Read the model definition and answer for the solid it produces. Units are mm, in the model's axes. Face numbers are marked on the shaded views. Round coordinates to 2 decimals unless told otherwise and drop trailing zeros.
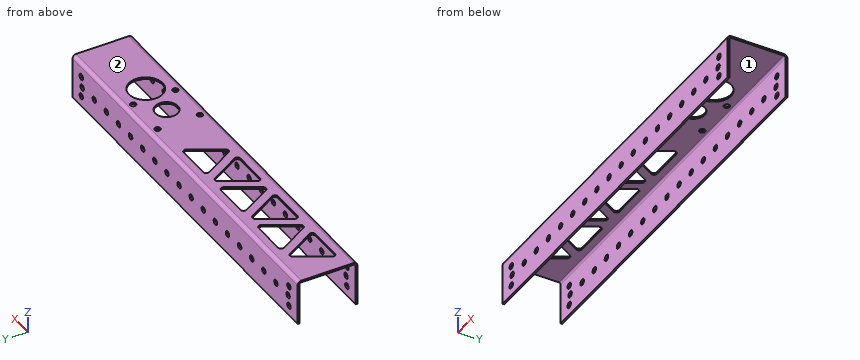
from build123d import *

# Parameters (mm, degrees)
BASE_FLANGE2_DEPTH = 165.1
SKETCH10_R         = 2.54
CUT_EXTRUDE1_DEPTH = 174.785938729
SKETCH11_R         = 14.2875
SKETCH11_R_2       = 9.525
SKETCH11_R_3       = 2.413
CUT_EXTRUDE2_DEPTH = 172.332367053
CUT_EXTRUDE3_DEPTH = 2.54
SKETCH13_R         = 2.54
CUT_EXTRUDE4_DEPTH = 174.785938729


# Sheet-metal steps are written as plain solids
with BuildPart() as part:
    # Sketch1 → Base-Flange2 (new, symmetric)
    with BuildSketch(Plane(origin=(0, 0, 0), x_dir=(0, 0, -1), z_dir=(1, 0, 0))):
        with BuildLine():
            Line((19.05, -25.4), (-15.875, -25.4))
            ThreePointArc((-15.875, -25.4), (-18.12006403, -24.47006403), (-19.05, -22.225))
            Line((-19.05, -22.225), (-19.05, 22.225))
            ThreePointArc((-19.05, 22.225), (-18.12006403, 24.47006403), (-15.875, 25.4))
            Line((-15.875, 25.4), (19.05, 25.4))
            Line((19.05, 25.4), (19.05, 23.8125))
            Line((19.05, 23.8125), (-15.875, 23.8125))
            ThreePointArc((-15.875, 23.8125), (-16.997532015, 23.347532015), (-17.4625, 22.225))
            Line((-17.4625, 22.225), (-17.4625, -22.225))
            ThreePointArc((-17.4625, -22.225), (-16.997532015, -23.347532015), (-15.875, -23.8125))
            Line((-15.875, -23.8125), (19.05, -23.8125))
            Line((19.05, -23.8125), (19.05, -25.4))
        make_face()
    extrude(amount=BASE_FLANGE2_DEPTH, both=True)

    # Sketch10 → Cut-Extrude1 (cut, through all)
    with BuildSketch(Plane(origin=(0, 25.4, 0), x_dir=(1, 0, 0), z_dir=(0, 1, 0))):
        with Locations(Location((151.13, 1.5875, 0), (0, 0, 270))):
            Circle(SKETCH10_R)
        with Locations(Location((133.35, 1.5875, 0), (0, 0, 270))):
            Circle(SKETCH10_R)
        with Locations(Location((115.57, 1.5875, 0), (0, 0, 270))):
            Circle(SKETCH10_R)
        with Locations(Location((97.79, 1.5875, 0), (0, 0, 270))):
            Circle(SKETCH10_R)
        with Locations(Location((80.01, 1.5875, 0), (0, 0, 270))):
            Circle(SKETCH10_R)
        with Locations(Location((62.23, 1.5875, 0), (0, 0, 270))):
            Circle(SKETCH10_R)
        with Locations(Location((44.45, 1.5875, 0), (0, 0, 270))):
            Circle(SKETCH10_R)
        with Locations(Location((26.67, 1.5875, 0), (0, 0, 270))):
            Circle(SKETCH10_R)
        with Locations(Location((8.89, 1.5875, 0), (0, 0, 270))):
            Circle(SKETCH10_R)
        with Locations(Location((-8.89, 1.5875, 0), (0, 0, 270))):
            Circle(SKETCH10_R)
        with Locations(Location((-26.67, 1.5875, 0), (0, 0, 270))):
            Circle(SKETCH10_R)
        with Locations(Location((-44.45, 1.5875, 0), (0, 0, 270))):
            Circle(SKETCH10_R)
        with Locations(Location((-62.23, 1.5875, 0), (0, 0, 270))):
            Circle(SKETCH10_R)
        with Locations(Location((-80.01, 1.5875, 0), (0, 0, 270))):
            Circle(SKETCH10_R)
        with Locations(Location((-97.79, 1.5875, 0), (0, 0, 270))):
            Circle(SKETCH10_R)
        with Locations(Location((-115.57, 1.5875, 0), (0, 0, 270))):
            Circle(SKETCH10_R)
        with Locations(Location((-133.35, 1.5875, 0), (0, 0, 270))):
            Circle(SKETCH10_R)
        with Locations(Location((-151.13, 1.5875, 0), (0, 0, 270))):
            Circle(SKETCH10_R)
    extrude(amount=-CUT_EXTRUDE1_DEPTH, mode=Mode.SUBTRACT)

    # Sketch11 → Cut-Extrude2 (cut, through all)
    with BuildSketch(Plane.XY.offset(19.05)):
        with Locations((101.6, 0)):
            Circle(SKETCH11_R)
        with Locations((71.12, 0)):
            Circle(SKETCH11_R_2)
        with Locations((53.159487758, 17.960512242)):
            Circle(SKETCH11_R_3)
        with Locations((89.080512242, 17.960512242)):
            Circle(SKETCH11_R_3)
        with Locations((89.080512242, -17.960512242)):
            Circle(SKETCH11_R_3)
        with Locations((53.159487758, -17.960512242)):
            Circle(SKETCH11_R_3)
    extrude(amount=-CUT_EXTRUDE2_DEPTH, mode=Mode.SUBTRACT)

    # Sketch12 → Cut-Extrude3 (cut)
    with BuildSketch(Plane.XY.offset(19.05)):
        with BuildLine():
            Line((-135.902216058, 12.3825), (-150.200295474, -12.3825))
            ThreePointArc((-150.200295474, -12.3825), (-150.200295474, -14.9225), (-148.000590949, -16.1925))
            Line((-148.000590949, -16.1925), (-119.404432116, -16.1925))
            ThreePointArc((-119.404432116, -16.1925), (-117.20472759, -14.9225), (-117.20472759, -12.3825))
            Line((-117.20472759, -12.3825), (-131.502807007, 12.3825))
            ThreePointArc((-131.502807007, 12.3825), (-133.702511532, 13.6525), (-135.902216058, 12.3825))
        make_face()
        with BuildLine():
            Line((-120.504284379, 16.1925), (-91.908125546, 16.1925))
            ThreePointArc((-91.908125546, 16.1925), (-89.70842102, 14.9225), (-89.70842102, 12.3825))
            Line((-89.70842102, 12.3825), (-104.006500437, -12.3825))
            ThreePointArc((-104.006500437, -12.3825), (-106.206204962, -13.6525), (-108.405909488, -12.3825))
            Line((-108.405909488, -12.3825), (-122.703988904, 12.3825))
            ThreePointArc((-122.703988904, 12.3825), (-122.703988904, 14.9225), (-120.504284379, 16.1925))
        make_face()
        with BuildLine():
            Line((-80.909602918, 12.3825), (-95.207682334, -12.3825))
            ThreePointArc((-95.207682334, -12.3825), (-95.207682334, -14.9225), (-93.007977808, -16.1925))
            Line((-93.007977808, -16.1925), (-64.411818976, -16.1925))
            ThreePointArc((-64.411818976, -16.1925), (-62.21211445, -14.9225), (-62.21211445, -12.3825))
            Line((-62.21211445, -12.3825), (-76.510193866, 12.3825))
            ThreePointArc((-76.510193866, 12.3825), (-78.709898392, 13.6525), (-80.909602918, 12.3825))
        make_face()
        with BuildLine():
            Line((-65.511671238, 16.1925), (-36.915512405, 16.1925))
            ThreePointArc((-36.915512405, 16.1925), (-34.71580788, 14.9225), (-34.71580788, 12.3825))
            Line((-34.71580788, 12.3825), (-49.013887296, -12.3825))
            ThreePointArc((-49.013887296, -12.3825), (-51.213591822, -13.6525), (-53.413296347, -12.3825))
            Line((-53.413296347, -12.3825), (-67.711375764, 12.3825))
            ThreePointArc((-67.711375764, 12.3825), (-67.711375764, 14.9225), (-65.511671238, 16.1925))
        make_face()
        with BuildLine():
            Line((-25.916989777, 12.3825), (-40.215069194, -12.3825))
            ThreePointArc((-40.215069194, -12.3825), (-40.215069194, -14.9225), (-38.015364668, -16.1925))
            Line((-38.015364668, -16.1925), (-9.419205835, -16.1925))
            ThreePointArc((-9.419205835, -16.1925), (-7.21950131, -14.9225), (-7.21950131, -12.3825))
            Line((-7.21950131, -12.3825), (-21.517580726, 12.3825))
            ThreePointArc((-21.517580726, 12.3825), (-23.717285252, 13.6525), (-25.916989777, 12.3825))
        make_face()
        with BuildLine():
            Line((-10.519058098, 16.1925), (18.077100735, 16.1925))
            ThreePointArc((18.077100735, 16.1925), (20.276805261, 14.9225), (20.276805261, 12.3825))
            Line((20.276805261, 12.3825), (5.978725844, -12.3825))
            ThreePointArc((5.978725844, -12.3825), (3.779021318, -13.6525), (1.579316793, -12.3825))
            Line((1.579316793, -12.3825), (-12.718762624, 12.3825))
            ThreePointArc((-12.718762624, 12.3825), (-12.718762624, 14.9225), (-10.519058098, 16.1925))
        make_face()
    extrude(amount=-CUT_EXTRUDE3_DEPTH, mode=Mode.SUBTRACT)

    # Sketch13 → Cut-Extrude4 (cut, through all)
    with BuildSketch(Plane(origin=(0, 25.4, 0), x_dir=(1, 0, 0), z_dir=(0, 1, 0))):
        with Locations(Location((-152.4, 10.31875, 0), (0, 0, 270))):
            Circle(SKETCH13_R)
        with Locations(Location((-152.4, -7.14375, 0), (0, 0, 270))):
            Circle(SKETCH13_R)
        with Locations(Location((152.4, -7.14375, 0), (0, 0, 270))):
            Circle(SKETCH13_R)
        with Locations(Location((152.4, 10.31875, 0), (0, 0, 270))):
            Circle(SKETCH13_R)
    extrude(amount=-CUT_EXTRUDE4_DEPTH, mode=Mode.SUBTRACT)


solid = part.part
Q1. Determine the mould class of the marked faces 1 and 2 for opening direction Y: pulls with the +Y half, pulls with the -Y half, needs draft (parallel to the pull), parting line crosses it, or undercut.
Verdict:
face 1: undercut
face 2: needs draft
Q2. Section B-B (y = 3.5) is taken. State how many separate pieces and enclosed holes the cut face has, then the cut area to 3 significant figures.
Verdict:
separate pieces: 9
enclosed holes: 0
area: 274 mm2
Q3. Flat-ended cylindrical pins translate along their axes: pin 1 Ø4 at (x, z) = (-151.13, -1.59) entering from -Y; pin 2 Ø6 at (x, z) = (44.45, -1.59) entering from +Y; pin 3 Ø1.3 at (x, z) = (-131, 18) entering from +Y; pin 4 Ø4 at (x, y) = (-67.5, 18.5) entering from -Z. Find the tip coordinate at first contact, or state that the pin passes through.
Verdict:
pin 1: passes through
pin 2: stops at y = 25.4
pin 3: stops at y = 25.04
pin 4: stops at z = 17.46
Q4. Straight lines are drawn through the part: probe 1 along Y at (x, z) = (-94.5, -16); probe 2 along Z at (x, y) = (145.5, 15.5); probe 3 along Y at (x, z) = (101.6, 18.05). For each, find the intervals that lie inside material, in ascending order.
Verdict:
probe 1: y = -25.4 to -23.81, 23.81 to 25.4
probe 2: z = 17.46 to 19.05
probe 3: y = -24.54 to -14.29, 14.29 to 24.54
